```python
from build123d import *

# Parameters (mm, degrees)
SKETCH1_R           = 2.1
BOSS_EXTRUDE1_DEPTH = 1
SKETCH2_R           = 1.5
BOSS_EXTRUDE2_DEPTH = 50
SKETCH3_R           = 2.1
BOSS_EXTRUDE3_DEPTH = 1
FILLET1_R           = 1


with BuildPart() as part:
    # Sketch1 → Boss-Extrude1 (new body)
    with BuildSketch(Plane(origin=(0, 0, 0), x_dir=(0, 0, -1), z_dir=(1, 0, 0))):
        Circle(SKETCH1_R)
    extrude(amount=BOSS_EXTRUDE1_DEPTH)

    # Sketch2 → Boss-Extrude2 (add)
    with BuildSketch(Plane(origin=(1, 0, 0), x_dir=(0, 0, -1), z_dir=(1, 0, 0))):
        Circle(SKETCH2_R)
    extrude(amount=BOSS_EXTRUDE2_DEPTH)

    # Sketch3 → Boss-Extrude3 (add)
    with BuildSketch(Plane(origin=(51, 0, 0), x_dir=(0, 0, -1), z_dir=(1, 0, 0))):
        Circle(SKETCH3_R)
    extrude(amount=BOSS_EXTRUDE3_DEPTH)

    # Fillet1
    fillet1_edges = [part.edges().sort_by_distance(p)[0] for p in [
        (0, 0, 2.1),
        (52, 0, 2.1),
    ]]
    fillet(fillet1_edges, radius=FILLET1_R - 0.0001)  # a hair under: the kernel refuses the full size


solid = part.part
```
Here's how the part is built. I have some questions about the finished solid (model axes, mm). Coordinates: 2 decimals unless noted, no trailing zeros. Write each loop counter-clockwise with the first axis right and the second up, starting at its lowest first coordinate (ties: lowest second). Pieces come first, ordered by that corner, then holes. Notation, with made-up numbers: (-21.5, -5.5) -> (-3.5, -5.5) arc R37 ccw to (-3.5, 31.5) -> close; hole circle Ø5 at (61.5, 56). An arc over 180 degrees is marked (long way). Use a Markdown table: item, result. Add a question column.
(1) If we section it at C-C, the plane x = 27.5: Write out the boundary of the cut face in (y, z), and give its area (3 significant figures).
(2) We'd pull the mould along X, two halves only. Please class faces 1 (the flat face through (0, 0, 0)), 2 (the flat face through (52, 0, 0)), 3 (the flat face through (1, -0.9, -1.4)): +X half, -X half, draft (parallel to the pull), parting line (faces both ways), or undercut.
(3) I'm going to push flat-ended pins straight in: P1, Ø1, axis at x = 32, z = -0.5, coming from the +Y side; P2, Ø2, axis at x = 39.5, y = -1, coming from the +Z side. Where does each tip first touch, or does it pass through?
(4) Please list where these lines run through material, in increasing order: line 1 (X direction, y = 1.25, z = -0.9); line 2 (X direction, y = 1.45, z = -1); line 3 (Z direction, x = 41, y = 0.1).
Outcome:
| question | item | result |
|---|---|---|
| 1 | outline | circle Ø3 at (0, 0) |
| 1 | area | 7.07 mm^2 |
| 2 | face 1 | -X half |
| 2 | face 2 | +X half |
| 2 | face 3 | undercut |
| 3 | P1 | stops at y = 1.5 |
| 3 | P2 | stops at z = 1.5 |
| 4 | line 1 | x = 0.1 to 1, 51 to 51.9 |
| 4 | line 2 | x = 0.25 to 1, 51 to 51.75 |
| 4 | line 3 | z = -1.5 to 1.5 |
